Verification items for the finished model (mm, model axes). Face numbers are marked on the shaded views. A direction names the side the tool comes from. Round coordinates to 2 decimals unless told otherwise and drop trailing zeros. Write each loop counter-clockwise with the first axis right and the second up, starting at its lowest first coordinate (ties: lowest second). Pieces come first, ordered by that corner, then holes.
from build123d import *

# Parameters (mm, degrees)
F1_DEPTH = 203.2
F2_R     = 5.08
F3_W     = 15.24
F3_H     = 50.8
F4_DEPTH = 3.9456780069
F5_R     = 7.61999
F6_W     = 15.24
F6_H     = 38.1
F7_DEPTH = 4.1115754284
F8_R     = 7.61999


# Not quite as in the source:
# - a fillet or chamfer is up to 0.001 mm smaller than in the source, because OpenCascade refuses the exact size


with BuildPart() as f1:
    # F0 (on Front) → F1 (new body)
    with BuildSketch(Plane.XZ):
        Polygon((59.1770336032, 0), (0, 0), (0, 111.0939458013), (-3.9456780069, 111.0939458013), (-3.9456780069, -4.1115754284), (59.1770336032, -4.1115754284), align=None)
    extrude(amount=F1_DEPTH)

    # F2
    f2_edges = [f1.edges().sort_by_distance(p)[0] for p in [
        (-1.972839, -203.2, 111.093946),
        (59.177034, -203.2, -2.055788),
        (59.177034, 0, -2.055788),
        (-1.972839, 0, 111.093946),
    ]]
    fillet(f2_edges, radius=F2_R)

    # F3 (on face) → F4 (cut, through all)
    with BuildSketch(Plane.YZ):
        with Locations((-170.18, 60.2939458013)):
            Rectangle(F3_W, F3_H)
        with Locations((-33.02, 60.2939458013)):
            Rectangle(F3_W, F3_H)
    extrude(amount=-F4_DEPTH, mode=Mode.SUBTRACT)

    # F5 (radius 7.62 in the source; OpenCascade refuses exactly that, so slightly less here)
    f5_edges = [f1.edges().sort_by_distance(p)[0] for p in [
        (-1.972839, -177.8, 34.893946),
        (-1.972839, -162.56, 34.893946),
        (-1.972839, -177.8, 85.693946),
        (-1.972839, -162.56, 85.693946),
        (-1.972839, -40.64, 85.693946),
        (-1.972839, -25.4, 85.693946),
        (-1.972839, -40.64, 34.893946),
        (-1.972839, -25.4, 34.893946),
    ]]
    fillet(f5_edges, radius=F5_R)

    # F6 (on face) → F7 (cut, through all)
    with BuildSketch(Plane.XY):
        with Locations((38.8570336032, -146.05)):
            Rectangle(F6_W, F6_H)
        with Locations((38.8570336032, -57.15)):
            Rectangle(F6_W, F6_H)
    extrude(amount=-F7_DEPTH, mode=Mode.SUBTRACT)

    # F8 (radius 7.62 in the source; OpenCascade refuses exactly that, so slightly less here)
    f8_edges = [f1.edges().sort_by_distance(p)[0] for p in [
        (31.237034, -165.1, -2.055788),
        (46.477034, -165.1, -2.055788),
        (31.237034, -127, -2.055788),
        (46.477034, -127, -2.055788),
        (46.477034, -38.1, -2.055788),
        (46.477034, -76.2, -2.055788),
        (31.237034, -76.2, -2.055788),
        (31.237034, -38.1, -2.055788),
    ]]
    fillet(f8_edges, radius=F8_R)


solid = f1.part
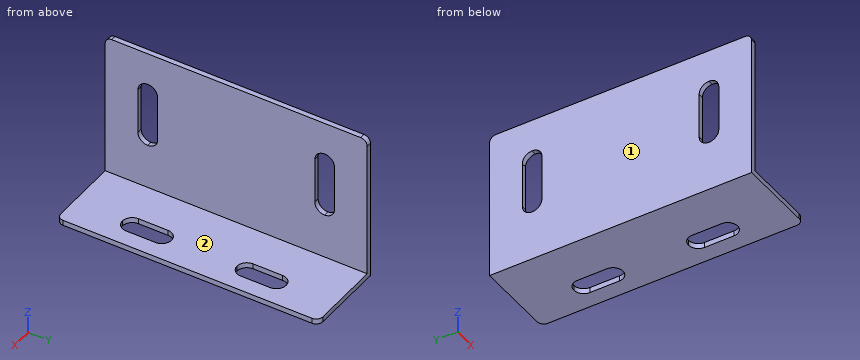
Q1. Material ranges on line 1 along X through (y, z) = (-86.5, 27.5); line 2 along Z through (x, y) = (2, -180), recorded low to high.
Recorded:
line 1: x = -3.95 to 0
line 2: z = -4.11 to 0
Q2. Tool access check on the marked faces 1 and 2. Record the directions out of +Z, -Z, +X, -X, +Y, -Y that give a thin tool (end or side, any length) a straight path to the whole face; none if there is none.
Recorded:
face 1: +Z, -Z, -X, +Y, -Y
face 2: +Z, +X, +Y, -Y
Q3. Sectioned sample at B-B (y = -80.5). Enter the section's corners in (x, z), plus the area to 3 significant figures.
Recorded:
outline: (-3.95, -4.11) - (59.18, -4.11) - (59.18, 0) - (0, 0) - (0, 111.09) - (-3.95, 111.09) - close
area: 698 mm2
Q4. Sectioned sample at D-D (z = 24). Enter the section's corners in (x, y), plus the area to 3 significant figures.
Recorded:
outline: (-3.95, -203.2) - (0, -203.2) - (0, 0) - (-3.95, 0) - close
area: 802 mm2
Q5. Depth check by flat-ended pin: P1, Ø10, axis at x = 42, y = -90, coming from the +Z side; P2, Ø1, axis at y = -74, z = 54.5, coming from the +X side. Enter the tip coordinate at first touch or a pass-through.
Recorded:
P1: stops at z = 0
P2: stops at x = 0
Q6. Sectioned sample at C-C (x = 50). Enter the section's corners in (y, z).
Recorded:
outline: (-203.2, -4.11) - (0, -4.11) - (0, 0) - (-203.2, 0) - close
Q7. Sectioned sample at A-A (z = 57.5). Enter the section's corners in (x, y).
Recorded:
outline: (-3.95, -203.2) - (0, -203.2) - (0, -177.8) - (-3.95, -177.8) - close; (-3.95, -162.56) - (0, -162.56) - (0, -40.64) - (-3.95, -40.64) - close; (-3.95, -25.4) - (0, -25.4) - (0, 0) - (-3.95, 0) - close
